```python
from build123d import *

# Parameters (mm, degrees)
BOSS_EXTRUDE1_DEPTH  = 6.5
BOSS_EXTRUDE2_DEPTH  = 3
M4_CLEARANCE_HOLE1_D = 4.3


with BuildPart() as part:
    # Sketch2 → Boss-Extrude1 (new body)
    with BuildSketch(Plane.XY):
        with BuildLine():
            Line((-49.497947743, 4.45), (-36.897947743, 4.45))
            ThreePointArc((-36.897947743, 4.45), (-34.447947743, 2), (-36.897947743, -0.45))
            Line((-36.897947743, -0.45), (-49.497947743, -0.45))
            ThreePointArc((-49.497947743, -0.45), (-51.947947743, 2), (-49.497947743, 4.45))
        make_face()
    extrude(amount=-BOSS_EXTRUDE1_DEPTH)

    # Sketch3 → Boss-Extrude2 (add)
    with BuildSketch(Plane.XY):
        with BuildLine():
            Line((-49.497947743, 6.5), (-36.897947743, 6.5))
            ThreePointArc((-36.897947743, 6.5), (-32.397947743, 2), (-36.897947743, -2.5))
            Line((-36.897947743, -2.5), (-49.497947743, -2.5))
            ThreePointArc((-49.497947743, -2.5), (-53.997947743, 2), (-49.497947743, 6.5))
        make_face()
    extrude(amount=BOSS_EXTRUDE2_DEPTH)

    # M4 Clearance Hole1 (through all)
    with Locations(Plane(origin=(-47.697947743, 2, 3), x_dir=(1, 0, 0), z_dir=(0, 0, 1))):
        with Locations((0, 0), (10, 0)):
            Hole(M4_CLEARANCE_HOLE1_D / 2)


solid = part.part
```
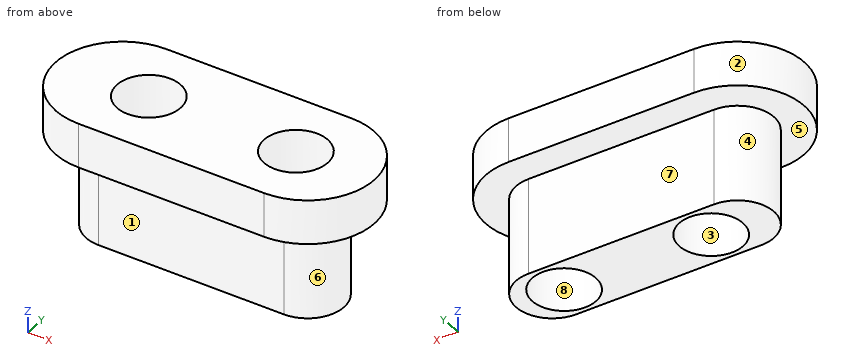
CAD build for the part. Positions are in the model's coordinates, mm. Face numbers are marked on the shaded views. A direction names the side the tool comes from. Round coordinates to 2 decimals unless told otherwise and drop trailing zeros. Order: outer loops, then holes, each group sorted by start corner. A loop starts at its lowest first (then second) coordinate and runs counter-clockwise, first axis right, second up. Notation, with made-up numbers: (45.5, -37) - (72.5, -37) arc R26 ccw to (72.5, -15) - close; hole circle Ø10 at (54.25, 67.25). An arc over 180 degrees is marked (long way). Answer as CSV lines item,"result". Start each with the question number.
1. Saw through at C-C, the plane x = -40.25. Write the cut outline in (y, z), and give its area (4 significant figures).
2. Saw through at A-A, the plane y = 2. Write the cut outline in (x, z), and give its area (4 significant figures).
3. Saw through at D-D, the plane y = 3.75. Write the cut outline in (x, z).
4. Pin check, flat tips, straight feed: pin 1 (3 mm diameter, centred on y = 3.5, z = -5.5, fed in from +X); pin 2 (2 mm diameter, centred on y = -1, z = 0, fed in from +X); pin 3 (2 mm diameter, centred on x = -46, z = -3.5, fed in from +Y); pin 4 (3.5 mm diameter, centred on x = -47.7, y = 2, fed in from +Z). Stop position of each tip, or through.
5. Pull direction X, two halves, no side cores. Call the marked faces 1, 2 and 3: +X half, -X half, draft (parallel to the pull), parting line (faces both ways), or undercut.
6. Tool access for the marked faces 4, 5, 6, 7 and 8: list every direction of +Z, -Z, +X, -X, +Y, -Y with a clear straight run to the whole face (end or side of a thin tool).
7. Drill centre lines: L1, parallel to X at y = 0.25, z = -5; L2, parallel to Y at x = -43.5, z = -0.5; L3, parallel to Z at x = -47.5, y = 5.5. Where is each one in solid material? Low to high. Write a range as [from, to].
8. Saw through at B-B, the plane z = -2.25. Write the cut outline in (x, y), and give its area (3 significant figures).
Model answer:
1,outline,"(-2.5, 0) - (-0.45, 0) - (-0.45, -6.5) - (4.45, -6.5) - (4.45, 0) - (6.5, 0) - (6.5, 3) - (-2.5, 3) - close"
1,area,"58.85 mm²"
2,outline,"(-54, 0) - (-51.95, 0) - (-51.95, -6.5) - (-49.85, -6.5) - (-49.85, 3) - (-54, 3) - close; (-45.55, -6.5) - (-39.85, -6.5) - (-39.85, 3) - (-45.55, 3) - close; (-35.55, -6.5) - (-34.45, -6.5) - (-34.45, 0) - (-32.4, 0) - (-32.4, 3) - (-35.55, 3) - close"
2,area,"96.85 mm²"
3,outline,"(-53.64, 0) - (-51.21, 0) - (-51.21, -6.5) - (-48.95, -6.5) - (-48.95, 3) - (-53.64, 3) - close; (-46.45, -6.5) - (-38.95, -6.5) - (-38.95, 3) - (-46.45, 3) - close; (-36.45, -6.5) - (-35.18, -6.5) - (-35.18, 0) - (-32.75, 0) - (-32.75, 3) - (-36.45, 3) - close"
4,pin 1,"stops at x = -34.45"
4,pin 2,"stops at x = -32.87"
4,pin 3,"stops at y = 4.45"
4,pin 4,"passes through"
5,face 1,"draft"
5,face 2,"-X half"
5,face 3,"undercut"
6,face 4,"-Z, -X"
6,face 5,"-Z"
6,face 6,"-Z, +X"
6,face 7,"-Z, +X, -X, +Y"
6,face 8,"+Z, -Z"
7,L1,"x = [-51.21, -48.95], [-46.45, -38.95], [-36.45, -35.18]"
7,L2,"y = [-0.45, 4.45]"
7,L3,"z = [0, 3]"
8,outline,"(-49.5, -0.45) - (-36.9, -0.45) arc R2.45 ccw to (-36.9, 4.45) - (-49.5, 4.45) arc R2.45 ccw to start; hole circle Ø4.3 at (-47.7, 2); hole circle Ø4.3 at (-37.7, 2)"
8,area,"51.6 mm²"
